from build123d import *

# Parameters (mm, degrees)
F0_W     = 412.75
F0_H     = 88.9
F1_DEPTH = 12.7
F2_W     = 12.7
F2_H     = 25.4
F2_H_2   = 12.7
F3_DEPTH = 25.4
F4_W     = 12.7
F4_H     = 12.7
F5_DEPTH = 25.4
F6_W     = 12.7
F6_H     = 12.7
F7_DEPTH = 25.4


with BuildPart() as f1:
    # F0 (on Top) → F1 (new body)
    with BuildSketch(Plane.XY):
        with Locations((206.375, 44.45)):
            Rectangle(F0_W, F0_H)
    extrude(amount=F1_DEPTH)

    # F2 (on face) → F3 (cut)
    with BuildSketch(Plane.XY.offset(12.7)):
        with Locations((6.35, 12.7)):
            Rectangle(F2_W, F2_H)
        with Locations((6.35, 69.85)):
            Rectangle(F2_W, F2_H_2)
        with Locations((6.35, 44.45)):
            Rectangle(F2_W, F2_H_2)
    extrude(amount=-F3_DEPTH, mode=Mode.SUBTRACT)

    # F4 (on face) → F5 (cut)
    with BuildSketch(Plane.XY.offset(12.7)):
        with Locations((393.7, 6.35)):
            Rectangle(F4_W, F4_H)
        with Locations((368.3, 6.35)):
            Rectangle(F4_W, F4_H)
        with Locations((342.9, 6.35)):
            Rectangle(F4_W, F4_H)
    extrude(amount=-F5_DEPTH, mode=Mode.SUBTRACT)

    # F6 (on face) → F7 (cut)
    with BuildSketch(Plane.XY.offset(12.7)):
        with Locations((19.05, 6.35)):
            Rectangle(F6_W, F6_H)
        with Locations((44.45, 6.35)):
            Rectangle(F6_W, F6_H)
        with Locations((69.85, 6.35)):
            Rectangle(F6_W, F6_H)
    extrude(amount=-F7_DEPTH, mode=Mode.SUBTRACT)


solid = f1.part
Work out the finished part from the listing and answer in its coordinate system (mm). A direction names the side the tool comes from. Coordinates: 2 decimals unless noted, no trailing zeros. Loops run counter-clockwise (first coordinate to the right, second up) from the corner with the lowest first, then second, coordinate; pieces in that order, holes last. Notation, with made-up numbers: M 50,-33 L 63,-33 A32 ccw 63,-5 Z; hole C 27,9 d6. An arc over 180 degrees is marked long. Answer in a Markdown table with one row per item. Add a question column.
1. A tool of negligible diameter and unlimited length cuts with its end or side. For faces 1 (the flat face through (57, 0, 6)), 2 (the flat face through (19, 12.7, 6)), 3 (the flat face through (0, 82, 6)), 4 (the flat face through (70, 12.7, 6)), 5 (the flat face through (6, 38.1, 6)), from which of +Z, -Z, +X, -X, +Y, -Y can it reach the whole face along a straight path? Write none if from no direction.
2. Flat-ended cylindrical pins translate along their axes: P1, Ø4, axis at x = 4.5, z = 7.5, coming from the -Y side; P2, Ø4, axis at y = 7, z = 9, coming from the -X side; P3, Ø4, axis at x = 368.5, z = 6.5, coming from the -Y side. Find the tip coordinate at first contact, or state that the pin passes through.
3. The mould has two halves that part along X. Classify faces 6 (the flat face through (412.75, 44, 6)), 7 (the flat face through (203, 45, 0)), 8 (the flat face through (349.25, 6, 6)): pulls with the +X half, pulls with the -X half, needs draft (parallel to the pull), parting line crosses it, or undercut.
4. Find section A-A, the plane y = 45.5. Write down the section's boundary in (x, z).
5. Consider L1, parallel to X at y = 5.5, z = 8; L2, parallel to X at y = 50.5, z = 8; L3, parallel to Y at x = 70.5, z = 12.25. Determine where each line is inside the solid, lowest interval first.
Reported:
| question | item | result |
|---|---|---|
| 1 | face 1 | +Z, -Z, +X, -X, -Y |
| 1 | face 2 | +Z, -Z, -X, -Y |
| 1 | face 3 | +Z, -Z, -X, +Y, -Y |
| 1 | face 4 | +Z, -Z, -Y |
| 1 | face 5 | +Z, -Z, -X |
| 2 | P1 | stops at y = 25.4 |
| 2 | P2 | stops at x = 25.4 |
| 2 | P3 | stops at y = 12.7 |
| 3 | face 6 | pulls with the +X half |
| 3 | face 7 | needs draft |
| 3 | face 8 | undercut |
| 4 | outline | M 12.7,0 L 412.75,0 L 412.75,12.7 L 12.7,12.7 Z |
| 5 | L1 | x = 25.4 to 38.1, 50.8 to 63.5, 76.2 to 336.55, 349.25 to 361.95, 374.65 to 387.35, 400.05 to 412.75 |
| 5 | L2 | x = 12.7 to 412.75 |
| 5 | L3 | y = 12.7 to 88.9 |
